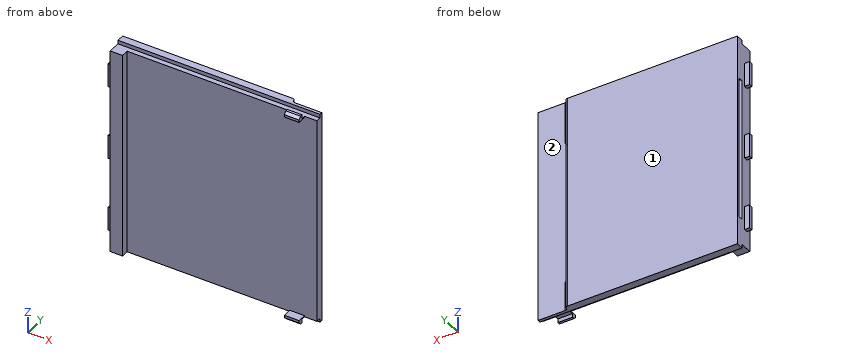
from build123d import *

# Parameters (mm, degrees)
SKETCH_2_W          = 87
SKETCH_2_H          = 3
SKETCH_2_W_2        = 2
SKETCH_2_H_2        = 2
SKETCH_2_W_3        = 80
EXTRUDE_1_DEPTH     = 82
SKETCH_3_W          = 84
SKETCH_3_H          = 8
EXTRUDE_2_DEPTH     = 5
SKETCH_3_3_W        = 9.6
SKETCH_3_3_H        = 1.5
EXTRUDE_3_DEPTH     = 2
SKETCH_4_W          = 58
SKETCH_4_H          = 0.8
CUT_EXTRUDE_1_DEPTH = 94.051061251
FILLET_1_R          = 1.2
CUT_EXTRUDE_START   = -0.3
CUT_EXTRUDE_2_DEPTH = 94.351061251
EXTRUDE_START       = 71
EXTRUDE_4_DEPTH     = 6
FILLET_2_R          = 1
FILLET_3_R          = 1


# Some blends are built 0.0001 mm under size
with BuildPart() as part:
    # Эскиз2 → Бобышка-Вытянуть1 (new body)
    with BuildSketch(Plane(origin=(0, 0, 0), x_dir=(0, 0, -1), z_dir=(1, 0, 0))):
        Rectangle(SKETCH_2_W, SKETCH_2_H)
        with Locations((-41, -2.5)):
            Rectangle(SKETCH_2_W_2, SKETCH_2_H_2)
        with Locations((41, -2.5)):
            Rectangle(SKETCH_2_W_2, SKETCH_2_H_2)
        with Locations((0, -2.5)):
            Rectangle(SKETCH_2_W_3, SKETCH_2_H_2)
    extrude(amount=EXTRUDE_1_DEPTH)

    # Эскиз3 → Бобышка-Вытянуть2 (add)
    with BuildSketch(Plane(origin=(0, 0, 0), x_dir=(0, 0, -1), z_dir=(1, 0, 0))):
        with Locations((0, -2.5)):
            Rectangle(SKETCH_3_W, SKETCH_3_H)
    extrude(amount=EXTRUDE_2_DEPTH)

    # Эскиз3<3> → Бобышка-Вытянуть3 (add)
    with BuildSketch(Plane(origin=(0, 0, 0), x_dir=(0, 0, -1), z_dir=(1, 0, 0))):
        with Locations((30, -3.9)):
            Rectangle(SKETCH_3_3_W, SKETCH_3_3_H)
        with Locations((0, -3.9)):
            Rectangle(SKETCH_3_3_W, SKETCH_3_3_H)
        with Locations((-30, -3.9)):
            Rectangle(SKETCH_3_3_W, SKETCH_3_3_H)
    extrude(amount=-EXTRUDE_3_DEPTH)

    # Эскиз4 → Вырез-Вытянуть1 (cut, through all)
    with BuildSketch(Plane(origin=(0, 0, 0), x_dir=(0, 0, -1), z_dir=(1, 0, 0))):
        with Locations((2.5, 0.1)):
            Rectangle(SKETCH_4_W, SKETCH_4_H)
    extrude(amount=CUT_EXTRUDE_1_DEPTH, mode=Mode.SUBTRACT)

    # Скругление1
    fillet_1_edges = [part.edges().sort_by_distance(p)[0] for p in [
        (0, -0.3, -2.5),
    ]]
    fillet(fillet_1_edges, radius=FILLET_1_R)

    # Эскиз5 → Вырез-Вытянуть2 (cut, through all)
    with BuildSketch(Plane(origin=(0, 0, 0), x_dir=(1, 0, 0), z_dir=(0, 1, 0)).offset(CUT_EXTRUDE_START)):
        Polygon((70, -47.531126979), (70, 0), (70, 45.964828752), (87.651611458, 45.964828752), (87.651611458, -47.531126979), align=None)
    extrude(amount=CUT_EXTRUDE_2_DEPTH, mode=Mode.SUBTRACT)

    # Эскиз6 → Бобышка-Вытянуть4 (add)
    with BuildSketch(Plane(origin=(0, 0, 0), x_dir=(0, 0, -1), z_dir=(1, 0, 0)).offset(EXTRUDE_START)):
        Polygon((-41.5, -3.049635954), (-42, -3.049635954), (-42, -5), (-43.5, -5), (-43.5, -6), (-42.5, -7), (-42, -7), (-41.5, -7), align=None)
    extrude_4 = extrude(amount=EXTRUDE_4_DEPTH)

    # Скругление2
    # the kernel refuses this fillet: 1 mm, written as the material it adds along each edge
    with BuildSketch(Plane(origin=(70, -0.3, 24), x_dir=(1, 0, 0), z_dir=(0, 0, 1))) as fillet_2_piece_1_section:
        with BuildLine():
            CenterArc((FILLET_2_R, FILLET_2_R), FILLET_2_R, 180, 90)
            Line((0, FILLET_2_R), (-FILLET_2_R * 0.02, FILLET_2_R))
            Line((-FILLET_2_R * 0.02, FILLET_2_R), (-FILLET_2_R * 0.02, -FILLET_2_R * 0.02))
            Line((-FILLET_2_R * 0.02, -FILLET_2_R * 0.02), (FILLET_2_R, -FILLET_2_R * 0.02))
            Line((FILLET_2_R, -FILLET_2_R * 0.02), (FILLET_2_R, 0))
        make_face()
    fillet_2_piece_1 = extrude(amount=19.5, mode=Mode.PRIVATE)
    fillet_2_piece_1 = split(fillet_2_piece_1, bisect_by=Plane(origin=(69.994030939, 0.5, 25.25), z_dir=(0, 1, 0)), keep=Keep.TOP, mode=Mode.PRIVATE)
    fillet_2_piece_1 = split(fillet_2_piece_1, bisect_by=Plane(origin=(69.994030939, 0.587417507, 26.5), z_dir=(0, 0, -1)), keep=Keep.TOP, mode=Mode.PRIVATE)
    with BuildSketch(Plane(origin=(70, -0.3, 26.5), x_dir=(1, 0, 0), z_dir=(0, 0, 1))) as fillet_2_piece_2_section:
        with BuildLine():
            CenterArc((FILLET_2_R, FILLET_2_R), FILLET_2_R, 180, 90)
            Line((0, FILLET_2_R), (-FILLET_2_R * 0.02, FILLET_2_R))
            Line((-FILLET_2_R * 0.02, FILLET_2_R), (-FILLET_2_R * 0.02, -FILLET_2_R * 0.02))
            Line((-FILLET_2_R * 0.02, -FILLET_2_R * 0.02), (FILLET_2_R, -FILLET_2_R * 0.02))
            Line((FILLET_2_R, -FILLET_2_R * 0.02), (FILLET_2_R, 0))
        make_face()
    fillet_2_piece_2 = extrude(amount=17, mode=Mode.PRIVATE)
    fillet_2_piece_2 = split(fillet_2_piece_2, bisect_by=Plane(origin=(70.231366514, 0.5, 35), z_dir=(0, -1, 0)), keep=Keep.TOP, mode=Mode.PRIVATE)
    with BuildSketch(Plane(origin=(70, -0.3, 26.5), x_dir=(1, 0, 0), z_dir=(0, 0, 1))) as fillet_2_piece_3_section:
        with BuildLine():
            CenterArc((FILLET_2_R, FILLET_2_R), FILLET_2_R, 180, 90)
            Line((0, FILLET_2_R), (-FILLET_2_R * 0.02, FILLET_2_R))
            Line((-FILLET_2_R * 0.02, FILLET_2_R), (-FILLET_2_R * 0.02, -FILLET_2_R * 0.02))
            Line((-FILLET_2_R * 0.02, -FILLET_2_R * 0.02), (FILLET_2_R, -FILLET_2_R * 0.02))
            Line((FILLET_2_R, -FILLET_2_R * 0.02), (FILLET_2_R, 0))
        make_face()
    fillet_2_piece_3 = extrude(amount=17, mode=Mode.PRIVATE)
    fillet_2_piece_3 = split(fillet_2_piece_3, bisect_by=Plane(origin=(69.994030939, 0.5, 35), z_dir=(0, 1, 0)), keep=Keep.TOP, mode=Mode.PRIVATE)
    add([fillet_2_piece_1, fillet_2_piece_2, fillet_2_piece_3])
    fillet_2_2_edges = [part.edges().sort_by_distance(p)[0] for p in [
        (70, -0.3, -37.5),
    ]]
    fillet(fillet_2_2_edges, radius=FILLET_2_R - 0.0001)  # a hair under: the kernel refuses the full size

    # Зеркальное отражение1: Бобышка-Вытянуть4 across plane
    add(extrude_4.mirror(Plane.XY))

    # Скругление3
    # the kernel refuses this fillet: 1 mm, written as the material it takes off along each edge
    with BuildSketch(Plane(origin=(70, 1.5, -45.974961047), x_dir=(0.005563569274726223, -0.9999845232286975, 0), z_dir=(0, 0, 1))) as fillet_3_piece_1:
        with BuildLine():
            CenterArc((0.994476676, -0.995532666), FILLET_3_R, 95.417808371, 84.263420946)
            Line((-0.005507847, -0.989969097), (-0.105506299, -0.98941274))
            Line((-0.105506299, -0.98941274), (-0.099998452, 0.000556357))
            Line((-0.099998452, 0.000556357), (0.000556357, 0.099998452))
            ThreePointArc((0.000556357, 0.099998452), (0.800643974, 0.095547041), (0.890617158, 0.099553267))
            Line((0.890617158, 0.099553267), (0.900058932, 0))
        make_face()
    fillet_3_piece_1_solid = extrude(amount=69.974960039, mode=Mode.PRIVATE)
    with BuildSketch(Plane(origin=(70, 1.5, 23.999998992), x_dir=(0.00556942794624549, -0.9999844906159053, 0), z_dir=(0, 0, 1))) as fillet_3_piece_2:
        with BuildLine():
            CenterArc((0.994470897, -0.995528948), FILLET_3_R, 95.420064112, 84.260829523)
            Line((-0.005513594, -0.98995952), (-0.105512043, -0.989402578))
            Line((-0.105512043, -0.989402578), (-0.099998449, 0.000556943))
            Line((-0.099998449, 0.000556943), (0.000556943, 0.099998449))
            ThreePointArc((0.000556943, 0.099998449), (0.800544535, 0.095542907), (0.890568265, 0.099552895))
            Line((0.890568265, 0.099552895), (0.900013959, 0))
        make_face()
    fillet_3_piece_2_solid = extrude(amount=21.974938193, mode=Mode.PRIVATE)
    add([fillet_3_piece_1_solid, fillet_3_piece_2_solid], mode=Mode.SUBTRACT)


solid = part.part
The model under review builds one solid part; all positions refer to its coordinate system, in mm. Face numbers are marked on the shaded views. Round coordinates to 2 decimals unless told otherwise and drop trailing zeros. Order: outer loops, then holes, each group sorted by start corner. A loop starts at its lowest first (then second) coordinate and runs counter-clockwise, first axis right, second up. Notation, with made-up numbers: (48.25, -7.5) -> (94.25, -7.5) arc R6 cw to (94.25, 3.5) -> close; hole circle Ø3 at (16, 2.5). An arc over 180 degrees is marked (long way). Use CSV: the item, a comma, the result in double quotes. Start each with the question number.
(1) Consider section B-B on x = 42.5. Write out the cut boundary in (y, z).
(2) Wall thickness on probe 1 along Y at (x, z) = (36.5, -4); probe 2 along X at (y, z) = (-2.75, 36.5); probe 3 along Z at (x, y) = (72.5, -2.75): over which ranges is each line inside the solid? List them lowest first. Write a range as from..to.
(3) Mouldability with a two-part tool opening along Z and no side actions: class the marked faces 1 and 2 as pulls with the +Z half, pulls with the -Z half, needs draft (parallel to the pull), parting line crosses it, or undercut.
(4) Consider section C-C on z = -1. Write out the cut boundary in (x, y) (3 decimals).
(5) Consider section D-D on z = -13. Write out the cut boundary in (x, y) (3 decimals), and give its area (3 significant figures).
(6) Consider section A-A on z = 29. Write out the cut boundary in (x, y).
(7) Insertion check: pin 1 (3 mm diameter, centred on y = -6, z = -31.5, fed in from +X); pin 2 (2.5 mm diameter, centred on x = 45, y = -5, fed in from -Z); pin 3 (1.5 mm diameter, centred on x = 55, y = -4, fed in from +Z); pin 4 (0.8 mm diameter, centred on x = -1, y = -3.5, fed in from +Z). Each pin has a flat end and moves straight along its axis. Give the tip position at first contact, or say it passes through.
Responses:
1,outline,"(-3.5, -42) -> (-1.5, -42) -> (-1.5, -43.5) -> (1.5, -43.5) -> (1.5, 43.5) -> (-1.5, 43.5) -> (-1.5, 42) -> (-3.5, 42) -> close; hole (-0.3, -31.5) -> (0.5, -31.5) -> (0.5, 26.5) -> (-0.3, 26.5) -> close"
2,probe 1,"-3.5..-0.3, 0.5..1.5"
2,probe 2,"0..82"
2,probe 3,"-42..42"
3,face 1,"needs draft"
3,face 2,"undercut"
4,outline,"(-2, -4.65) -> (0, -4.65) -> (0, -6.5) -> (5, -6.5) -> (5, -3.5) -> (82, -3.5) -> (82, -0.3) -> (1.2, -0.3) arc R1.2 ccw to (0, -1.5) -> (0, -3.15) -> (-2, -3.15) -> close; (0, 0.5) -> (70.02, 0.5) arc R1 cw to (70.005, 0.6) arc R1 ccw to (69.01, 1.5) -> (0, 1.5) -> close"
5,outline,"(0, -6.5) -> (5, -6.5) -> (5, -3.5) -> (82, -3.5) -> (82, -0.3) -> (1.2, -0.3) arc R1.2 ccw to (0, -1.5) -> close; (0, 0.5) -> (70.02, 0.5) arc R1 cw to (70.005, 0.6) arc R1 ccw to (69.01, 1.5) -> (0, 1.5) -> close"
5,area,"347 mm²"
6,outline,"(-2, -4.65) -> (0, -4.65) -> (0, -6.5) -> (5, -6.5) -> (5, -3.5) -> (82, -3.5) -> (82, -0.3) -> (71, -0.3) arc R1 cw to (70.01, 0.6) arc R1 ccw to (69.01, 1.5) -> (0, 1.5) -> (0, -3.15) -> (-2, -3.15) -> close"
7,pin 1,"x = 5"
7,pin 2,"through"
7,pin 3,"z = 42"
7,pin 4,"z = 34.8"
